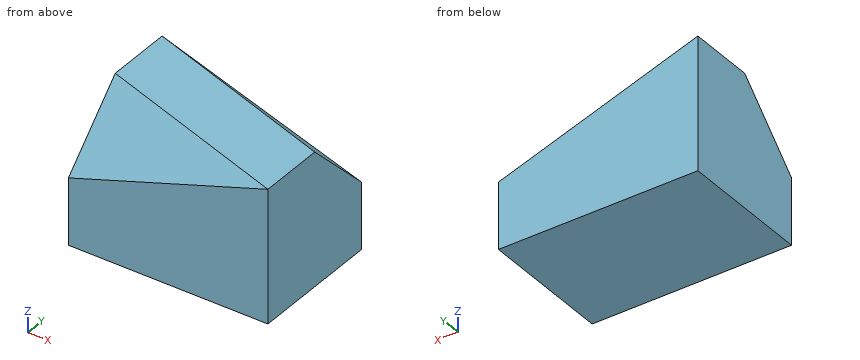
```python
from build123d import *

# Parameters (mm, degrees)
F0_W     = 60
F0_H     = 40
F1_DEPTH = 40
F5_DEPTH = 63.246553
F8_DEPTH = 63.246553


with BuildPart() as f1:
    # F0 (on Top) → F1 (new body)
    with BuildSketch(Plane.XY):
        with Locations((30, 20)):
            Rectangle(F0_W, F0_H)
    extrude(amount=F1_DEPTH)

    # F4 (on face) → F5 (cut, through all)
    with BuildSketch(Plane(origin=(-6, 2, 0), x_dir=(0.316228, 0.948683, 0), z_dir=(0.948683, -0.316228, 0))):
        Polygon((18.973666, 40), (0, 40), (0, 20), align=None)
    extrude(amount=F5_DEPTH, mode=Mode.SUBTRACT)

    # F7 (on face) → F8 (cut, through all)
    with BuildSketch(Plane(origin=(48, -16, 0), x_dir=(0.316228, 0.948683, 0), z_dir=(0.948683, -0.316228, 0))):
        Polygon((56.920998, 40), (37.947332, 40), (56.920998, 20), align=None)
    extrude(amount=-F8_DEPTH, mode=Mode.SUBTRACT)


solid = f1.part
```
Design review of the part built by this model. Coordinates are the model's own, in mm. Coordinates: 2 decimals unless noted, no trailing zeros. Write each loop counter-clockwise with the first axis right and the second up, starting at its lowest first coordinate (ties: lowest second). Pieces come first, ordered by that corner, then holes.
1) Add section D-D (y = 32). Write out the cut boundary in (x, z).
2) Add section B-B (z = 35). Write out the cut boundary in (x, y).
3) Add section C-C (y = 12.5). Write out the cut boundary in (x, z).
4) Insertion check: pin 1 (3 mm diameter, centred on x = 50, z = 34.5, fed in from +Y). The pin has a flat end and moves straight along its axis. Give the tip position at first contact, or say it passes through.
5) To check wall thickness, follow L1, parallel to Y at x = 23.5, z = 35; L2, parallel to Z at x = 15, y = 3; L3, parallel to Z at x = 18.5, y = 11. State the ranges of each line that lie inside material, in increasing order.
6) Add section A-A (x = 13). Write out the cut boundary in (y, z), plus the area to 3 significant figures.
Check result:
1. outline: (0, 0) - (60, 0) - (60, 28) - (24, 40) - (0, 40) - close
2. outline: (0, 15) - (45, 0) - (60, 0) - (60, 25) - (15, 40) - (0, 40) - close
3. outline: (0, 0) - (60, 0) - (60, 40) - (22.5, 40) - (0, 32.5) - close
4. pin 1: stops at y = 30.41
5. L1: y = 7.17 to 37.17
5. L2: z = 0 to 28
5. L3: z = 0 to 37.17
6. outline: (0, 0) - (40, 0) - (40, 35.67) - (35.67, 40) - (15.67, 40) - (0, 24.33) - close
6. area: 1,470 mm2
